The listing builds one solid part. Answer for the finished solid, in the listing's coordinates (mm). A direction names the side the tool comes from. Round coordinates to 2 decimals unless told otherwise and drop trailing zeros. Write each question's results on one line, items separated by ' | '. Start each with the question number.
from build123d import *

# Parameters (mm, degrees)
F0_R      = 12.7
F1_DEPTH  = 76.2
F1_FACE_R = 12.7
F2_DEPTH  = 25.4
F2_TAPER  = 30
F3_R      = 50.8
F4_T      = -2.54
F6_DEPTH  = 1.27
F7_SIZE   = 1.2699
F8_COUNT  = 3


# Not quite as in the source:
# - a fillet or chamfer is up to 0.001 mm smaller than in the source, because OpenCascade refuses the exact size


with BuildPart() as f1:
    # F0 (on Top) → F1 (new body)
    with BuildSketch(Plane.XY):
        Circle(F0_R)
    extrude(amount=F1_DEPTH)

    # F1_face (on face) → F2 (join)
    with BuildSketch(Plane.XY.offset(76.2)):
        Circle(F1_FACE_R)
    extrude(amount=F2_DEPTH, taper=F2_TAPER)

    # F3
    f3_edges = [f1.edges().sort_by_distance(p)[0] for p in [
        (-12.7, 0, 76.2),
    ]]
    fillet(f3_edges, radius=F3_R)

    # F4
    f4_openings = [f1.faces().sort_by_distance(p)[0] for p in [
        (0, 0, 0),
    ]]
    offset(amount=F4_T, openings=f4_openings)

    # F5 (on Right) → F6 (join, symmetric)
    with BuildSketch(Plane.YZ):
        Polygon((-36.83, 0), (-11.43, 0), (-11.43, 25.4), align=None)
    extrude(amount=F6_DEPTH, both=True)

    # F7 (size 1.27 in the source; OpenCascade refuses exactly that, so slightly less here)
    f7_edges = [f1.edges().sort_by_distance(p)[0] for p in [
        (1.27, -24.73317, 12.09683),
        (-1.27, -24.73317, 12.09683),
    ]]
    chamfer(f7_edges, length=F7_SIZE)

    # F8: F1 ×3 about axis
    f8_axis = Axis((0, 0, 0), (0, 0, 1))


with BuildPart() as f1_1:
    add(f1.part)
    for i in range(1, F8_COUNT):
        add(f1.part.rotate(f8_axis, i * 360 / F8_COUNT))


solid = f1_1.part
Item 1: For faces 1 (the flat face through (-1.27, -19, 6)), 2 (the flat face through (-15.832, 10.607, 6.378)), 3 (the cylindrical face through (-1.323, 10.074, 30.856)), determine the directions among +Z, -Z, +X, -X, +Y, -Y from which every point of the face is accessible in a straight line to the end or side of a thin tool.
Item 2: Straight lines are drawn through the part: L1, parallel to X at y = 0, z = 48; L2, parallel to Y at x = 9, z = 31. For each, find the intervals that lie inside material, in ascending order. Write a range as [from, to].
Item 3: Each of these flat-tipped pins is pushed along its axis until it touches: pin 1 Ø1.5 at (x, y) = (3.5, -25) entering from -Z; pin 2 Ø1.5 at (y, z) = (3, 31.5) entering from -X; pin 3 Ø6.5 at (y, z) = (-24.5, 9) entering from +X; pin 4 Ø4 at (y, z) = (7.5, 41) entering from -X. Where does it stop, or does it pass through?
Report:
1) face 1: +Z, -Z, -X, -Y | face 2: +Z, -Z, +Y | face 3: -Z
2) L1: x = [-12.7, -10.16], [10.16, 12.7] | L2: y = [-8.96, -4.71], [4.71, 8.96]
3) pin 1: passes through | pin 2: stops at x = -12.5 | pin 3: stops at x = 1.27 | pin 4: stops at x = -11.45
